```python
from build123d import *

# Parameters (mm, degrees)
F0_R     = 116.84
F0_W     = 107.95
F0_H     = 82.55
F1_DEPTH = 6.35
F3_DEPTH = 12.7


# Not quite as in the source:
# - ends of sketch curves that miss each other by under 0.0002 mm in the source are joined


with BuildPart() as f1:
    # F0 (on Front) → F1 (new body)
    with BuildSketch(Plane.XZ):
        Circle(F0_R)
        with BuildLine():
            ThreePointArc((57.9557025683, -82.6744686394), (0, -100.965), (-57.9557025683, -82.6744686394))
            ThreePointArc((-57.9557025683, -82.6744686394), (-63.2424676953, -74.0399131217), (-60.5362426444, -64.283798092))
            Line((-60.5362426444, -64.283798092), (-54.2551455528, -56.5256778711))
            ThreePointArc((-54.2551455528, -56.5256778711), (-49.8526531391, -53.0544887955), (-44.3845799964, -51.8170441872))
            Line((-44.3845799964, -51.8170441872), (44.3845799964, -51.8170441872))
            ThreePointArc((44.3845799964, -51.8170441872), (49.8526531391, -53.0544887955), (54.2551455528, -56.5256778711))
            Line((54.2551455528, -56.5256778711), (60.5362426444, -64.283798092))
            ThreePointArc((60.5362426444, -64.283798092), (63.2424676953, -74.0399131217), (57.9557025683, -82.6744686394))
        make_face(mode=Mode.SUBTRACT)
        Rectangle(F0_W, F0_H, mode=Mode.SUBTRACT)
    extrude(amount=F1_DEPTH)

    # F2 (on face) → F3 (cut, symmetric)
    with BuildSketch(Plane.XZ.offset(6.35)):
        Polygon((2.3792107569, 116.84), (-2.38125, 116.84), (-2.38125, 113.665), (2.3792661711, 113.665), align=None)
        Polygon((-2.38125, 113.665), (-2.38125, 116.84), (-2.3832892423, 116.8399584216), (-2.3832338281, 113.664958422), align=None)
        Polygon((2.38125, 116.84), (2.3792107569, 116.84), (2.3792661711, 113.6650415433), (2.38125, 113.665), align=None)
        Polygon((25.8521605942, 113.96895079), (21.1871487092, 114.9276323655), (20.5480276589, 111.8176244422), (25.2130395439, 110.8589428667), align=None)
        Polygon((48.2646865559, 106.4320251767), (43.8881478633, 108.3101400086), (42.6360713087, 105.3924475469), (47.0126100013, 103.514332715), align=None)
        Polygon((68.7012615192, 94.537784072), (64.7923710351, 97.2584423441), (62.9785988537, 94.6525153548), (66.8874893377, 91.9318570826), align=None)
        Polygon((86.3252143359, 78.7731764081), (83.0440016102, 82.2249946678), (80.742789437, 80.0375195173), (84.0240021628, 76.5857012576), align=None)
        Polygon((100.415022302, 59.7836035017), (97.8958198253, 63.8252646864), (95.2013790356, 62.1457963686), (97.7205815122, 58.1041351839), align=None)
        Polygon((110.3938502174, 38.3464963946), (108.7397938642, 42.8125353365), (105.7624345696, 41.709831101), (107.4164909228, 37.2437921591), align=None)
        Polygon((115.8531659566, 15.3394879114), (115.1319726134, 20.0470654638), (111.9935875785, 19.5662699016), (112.7147809217, 14.8586923493), align=None)
        Polygon((116.5694657294, -8.2955175322), (116.8106609728, -3.5391290804), (113.6397353383, -3.3783322514), (113.3985400948, -8.1347207032), align=None)
        Polygon((112.5134243011, -31.5909053937), (113.7071336244, -26.9804320664), (110.6334847395, -26.184625851), (109.4397754163, -30.7950991782), align=None)
        Polygon((103.8510955651, -53.5929650372), (105.9484486388, -49.3171591092), (103.0979113534, -47.9189237267), (101.0005582798, -52.1947296548), align=None)
        Polygon((90.9371143142, -73.4009345429), (93.8522457324, -69.6348470419), (91.3415207317, -67.6914260965), (88.4263893136, -71.4575135974), align=None)
        Polygon((74.3001775309, -90.2038778015), (77.9137421316, -87.1016919389), (75.8456182231, -84.6926488717), (72.2320536224, -87.7948347344), align=None)
        Polygon((54.6213995909, -103.3138841506), (58.7854584338, -101.0026030768), (57.2446043846, -98.2265638481), (53.0805455416, -100.537844922), align=None)
        Polygon((32.7064275147, -112.1942313615), (37.2505044854, -110.7684786712), (36.300002692, -107.7390940241), (31.7559257212, -109.1648467143), align=None)
        Polygon((9.4524578666, -116.4813589886), (14.1905189501, -115.9995048416), (13.869282852, -112.8407974526), (9.1312217685, -113.3226515996), align=None)
        Polygon((-14.1884943746, -115.9997524952), (-9.4504248819, -116.4815239474), (-9.1292439138, -113.3228109523), (-13.8673134065, -112.8410395), align=None)
        Polygon((-37.2485712051, -110.7691287983), (-32.704469351, -112.1948021792), (-31.7540204304, -109.1654009431), (-36.2981222845, -107.7397275622), align=None)
        Polygon((-58.7836955969, -101.0036290612), (-54.6195964151, -103.3148374582), (-53.0787908171, -100.538771337), (-57.2428899989, -98.22756294), align=None)
        Polygon((-77.9122219084, -87.1030517769), (-74.2986031649, -90.2051745705), (-72.2305213025, -87.7960954082), (-75.844140046, -84.6939726146), align=None)
        Polygon((-93.8510303607, -69.636485062), (-90.9358332124, -73.4025216837), (-88.4251421312, -71.4590569182), (-91.3403392796, -67.6930202964), align=None)
        Polygon((-105.9475878758, -49.3190082509), (-103.8501601756, -53.5947775726), (-100.9996472945, -52.1964924391), (-103.0970749947, -47.9207231174), align=None)
        Polygon((-113.7066627097, -26.9824166262), (-112.5128729187, -31.5928691186), (-109.4392379237, -30.797009258), (-110.6330277147, -26.1865567655), align=None)
        Polygon((-116.8105991856, -3.5411678105), (-116.5693209275, -8.2975520519), (-113.3983980999, -8.1366998799), (-113.639676358, -3.3803156385), align=None)
        Polygon((-115.1323224832, 20.0450560288), (-115.8534336636, 15.3374658899), (-112.7150402377, 14.856725103), (-111.9939290573, 19.5643152418), align=None)
        Polygon((-108.7405410673, 42.8106374625), (-110.3945194732, 38.3445696526), (-107.4171409332, 37.241917382), (-105.7631625274, 41.707985192), align=None)
        Polygon((-97.8969337715, 63.8235560723), (-100.4160657074, 59.7818509198), (-97.7215956058, 58.1024296292), (-95.2024636698, 62.1441347816), align=None)
        Polygon((-83.0454366945, 82.2235452641), (-86.3265891741, 78.7716697368), (-84.0253388226, 76.5842347504), (-80.744186343, 80.0361102776), align=None)
        Polygon((-64.7940685053, 97.2573114891), (-68.7029115043, 94.5365849944), (-66.8890938411, 91.9306896617), (-62.9802508421, 94.6514161565), align=None)
        Polygon((-43.8900382252, 108.3093739995), (-48.2665441378, 106.4311827828), (-47.0144166601, 103.5135121744), (-42.6379107474, 105.391703391), align=None)
        Polygon((-21.1891545716, 114.9272625625), (-25.8541497237, 113.9684995673), (-25.2149743936, 110.8585027993), (-20.5499792415, 111.8172657944), align=None)
    extrude(amount=F3_DEPTH, both=True, mode=Mode.SUBTRACT)


with BuildPart() as f4_1:
    # F4: copy of F1
    add(f1.part.moved(Location((0, 87.3125, 0))))


solid = f1.part
```
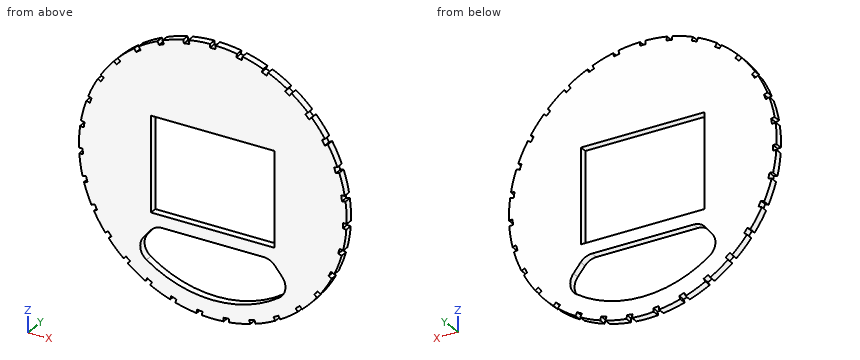
Work out the finished part from the listing and answer in its coordinate system (mm). Coordinates: 2 decimals unless noted, no trailing zeros. Loops run counter-clockwise (first coordinate to the right, second up) from the corner with the lowest first, then second, coordinate; pieces in that order, holes last.
1) Section A-A (y = -4.25) is taken. Give the number of separate pieces and of enclosed holes in the cut face, plus the area to 3 significant figures.
Results:
separate pieces: 1
enclosed holes: 2
area: 28,400 mm2
2) Section B-B (z = 52) is taken. Give the vertices of the cut face in (x, y).
Results:
outline: (-104.63, -6.35) - (104.63, -6.35) - (104.63, 0) - (-104.63, 0) - close
3) Flat-ended cylindrical pins translate along their axes: pin 1 (1.5 mm diameter, centred on x = -31, y = -2, fed in from -Z); pin 2 (1.9 mm diameter, centred on y = -3, z = -12.5, fed in from -X); pin 3 (1.5 mm diameter, centred on y = -3.5, z = 7, fed in from +X). Find the tip coordinate at first contact, or state that the pin passes through.
Results:
pin 1: stops at z = -112.86
pin 2: stops at x = -116.27
pin 3: stops at x = 116.67
4) Consider probe 1 along X at (y, z) = (-0.75, -85.5); probe 2 along Z at (x, y) = (-21.5, -0.25) (3 decimals); probe 3 along Z at (x, y) = (51, -3) (3 decimals). Determine where each line is inside the solid, lowest interval first.
Results:
probe 1: x = -79.63 to -76.54, -74.91 to -53.7, 53.7 to 74.91, 76.54 to 79.63
probe 2: z = -114.845 to -98.649, -51.817 to -41.275, 41.275 to 111.622
probe 3: z = -105.122 to -87.137, -53.676 to -41.275, 41.275 to 105.122
